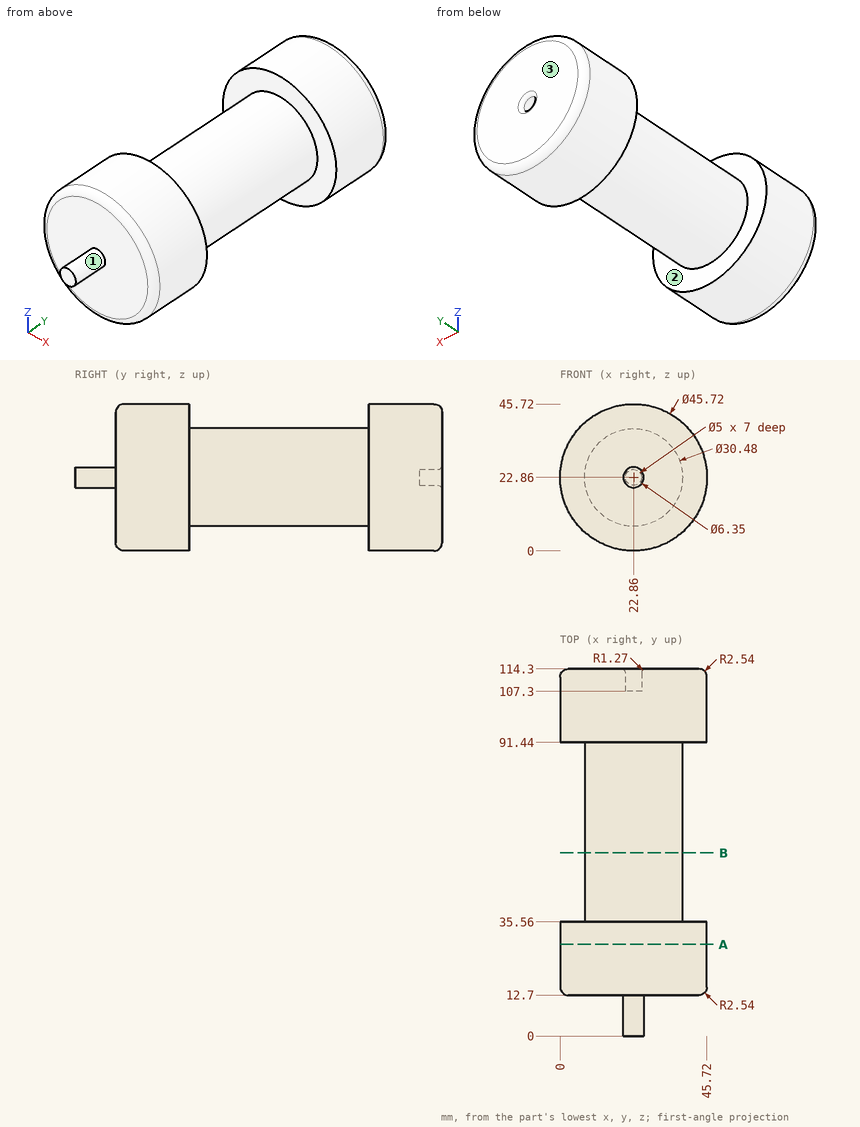
Can you work these out from the drawing? Everything is in mm from the part's minimum corner. A direction names the side the tool comes from. Coordinates: 2 decimals unless noted, no trailing zeros. Loops run counter-clockwise (first coordinate to the right, second up) from the corner with the lowest first, then second, coordinate; pieces in that order, holes last.
1) Please list where these lines run through material, in increasing order: line 1 along Y through (x, z) = (34.5, 10.5); line 2 along Y through (x, z) = (10.5, 23.5); line 3 along Z through (x, y) = (22, 111).
Reported:
line 1: y = 12.7 to 35.56, 91.44 to 114.3
line 2: y = 12.7 to 114.3
line 3: z = 0.02 to 20.51, 25.21 to 45.7
2) Will these pins go through, and if not, where does the flat tip stop? pin 1 Ø1 at (x, y) = (39, 82.5) entering from +Z; pin 2 Ø10 at (x, z) = (14.5, 33.5) entering from -Y; pin 3 Ø12 at (x, y) = (23, 76.5) entering from +Z; pin 4 Ø4 at (y, z) = (94, 14.5) entering from +X.
Reported:
pin 1: passes through
pin 2: stops at y = 12.7
pin 3: stops at z = 38.1
pin 4: stops at x = 44.82
3) Which directions (+Z, -Z, +X, -X, +Y, -Y) give clear straight access to the entire face, cutting with the end or side of a thin tool? Please do the marked faces 1, 2 and 3.
Reported:
face 1: -Y
face 2: none
face 3: +Z, -Z, +X, -X, +Y
4) Imagine slicing it at A-A (y = 28.5). List the corners of the cut face in (x, z) for me.
Reported:
outline: circle Ø45.72 at (22.86, 22.86)
5) Imagine slicing it at B-B (y = 57). List the corners of the cut face in (x, z) for me, and give its area (3 significant figures).
Reported:
outline: circle Ø30.48 at (22.86, 22.86)
area: 730 mm2
